Part model, mm, in its own coordinate system. A direction names the side the tool comes from. Round coordinates to 2 decimals unless told otherwise and drop trailing zeros. Loops run counter-clockwise (first coordinate to the right, second up) from the corner with the lowest first, then second, coordinate; pieces in that order, holes last.
1) Drop flat-ended pins along their axis: P1, Ø3, axis at x = 5, z = -2, coming from the -Y side; P2, Ø1, axis at x = 21, z = 2, coming from the +Y side; P3, Ø1.5, axis at x = 39.5, z = 3, coming from the -Y side. Give the stop position or say it passes through.
2) 3-axis set-ups, long thin cutter, end or side, ignore diameter. For faces 1 (the flat face through (-2.19, 0.99, -1.74)), 2 (the flat face through (50, 0, 0)): which of +Z, -Z, +X, -X, +Y, -Y reach the whole face in a straight line?
3) Probe line 1 (Z direction, x = 16.5, y = 0); line 2 (Y direction, x = 7, z = -1.25); line 3 (Y direction, x = 19, z = 2). List the from-to ranges inside material, lowest first.
4) Band-saw the part on A-A, the plane x = 36.5. Write the cut outline in (y, z).
5) Mould opens along Z. For faces 3 (the flat face through (-2, -2, 0)), 4 (the cylindrical face through (24, -3, 0)), 5 (the flat face through (0, -0.1, -3.4)), 6 (the flat face through (-2.186, 1.014, 1.724)) say: +Z half, -Z half, draft (parallel to the pull), parting line (faces both ways), or undercut.
Autodesk Inventor part; units mm, degrees
ref_plane "Work Plane1" through (29, 0, 0) normal (0, -1, 0) x (1, 0, 0)
ref_plane "YZ Plane" through (0, 0, 0) normal (1, 0, 0) x (0, 1, 0)
ref_plane "XZ Plane" through (0, 0, 0) normal (0, 1, 0) x (-1, 0, 0)
sketch "Sketch1" plane through (0, 0, 0) normal (0, 0, 1) x (1, 0, 0)
  line L0 (0.1133, 0) -> (50, 0)
  line L1 (50, 0) -> (50, 3)
  line L2 (50, 3) -> (26, 3)
  line L3 (26, 3) -> (25.3864, 3)
  line L4 (25.3864, 3) -> (0, 3)
  line L5 (0, 3) -> (0, 5.25)
  line L6 (0, 5.25) -> (-3.3, 5.25)
  line L7 (-3.3, 5.25) -> (-3.3, 2.3094)
  line L8 (-3.3, 2.3094) -> (-1.22, 2.3094)
  line L9 (-1.22, 2.3094) -> (0.1133, 0)
  line L10 (-13.96, 0) -> (60.66, 0)
  line L11 (0, -1.05) -> (0, 6.3)
  line L12 (26, 3) -> (0, 3) construction
  dimension "d1" = 24
  dimension "d2" = 0.6136
  dimension "d3" = 3.3
  dimension "d4" = 2.08
  dimension "d5" = 60
  dimension "d6" = 6
  dimension "d7" = 6
  dimension "d8" = 4.6188
  dimension "d9" = 10.5
  dimension "d26" = 50
revolve "Body" add sketch "Sketch1" angle 360 about axis through (0.1133, 0, 0) along (1, 0, 0) contours L9 L11 L4 L3 L2 L1 L0 | L9 L8 L7 L6 L5 L11
sketch "Sketch2" plane through (-3.3, 0, 0) normal (-1, 0, 0) x (0, 0, 1)
  circle A0 centre (0, 0) radius 2.3094
  line L0 (0, -7.35) -> (0, 7.35)
  line L1 (-7.35, 0) -> (7.35, 0)
  line L2 (2.3094, 0) -> (1.1547, -2)
  line L3 (1.1547, -2) -> (-1.1547, -2)
  line L4 (-1.1547, -2) -> (-2.3094, 0)
  line L5 (-2.3094, 0) -> (-1.1547, 2)
  line L6 (-1.1547, 2) -> (1.1547, 2)
  line L7 (1.1547, 2) -> (2.3094, 0)
extrude "Slot" add sketch "Sketch2" against normal up to next contours L7 A0 | A0 L2 | L6 L0 A0 | A0 L0 L3 | L0 L6 A0 | A0 L3 L0 | L4 A0 | A0 L5
fillet "Fillet1" radius 2.56 1 edges at (-3.3, -5.25, 0)
thread "Thread"
chamfer "Chamfer1" distance 0.6135 distance2 0.6135 1 edges at (50, -3, 0) measured on face at (50, -0.7485, -0.2663)
ref_plane "Work Plane1" through (29, 0, 0) normal (0, -1, 0) x (1, 0, 0)
fillet "Fillet2" radius 0.25 1 edges at (0, -3, 0)
equation "\"d1\" = GEL"
equation "\"d3\" = KOH"
equation "\"d4\" = INTI"
equation "\"d6\" = GD"
equation "\"d7\" = BDM"
equation "\"d8\" = 1.1547 * SW"
equation "\"d9\" = KOD"
equation "\"d26\" = NLG"
equation "\"d30\" = R"
equation "\"d17\" = RR"
equation "\"d13\" = GEL"
equation "\"d15\" = -0.5 * SPD + 0.5 * GD"
equation "\"d16\" = GUL"
equation "\"GD\" = NND"
equation "\"NLG\" = 50"
equation "\"GEL\" = 24"
equation "\"KOD\" = 10.5"
equation "\"KOH\" = 3.3"
equation "\"INTI\" = 2.08"
equation "\"GAL\" = 0.61345 * PTC"
equation "\"GUL\" = 0.61345 * PTC"
equation "\"BDM\" = NND"
equation "\"SW\" = 4"
equation "\"RR\" = 2.56"
equation "\"SPD\" = NND - 1.2269 * PTC"
equation "\"R\" = 0.25"
equation "\"TOA\" = 30deg"
equation "\"GD1\" = THREADDIA - 1.2269 * PTC"
equation "\"THREADDIA\" = 6"
equation "\"PTC\" = 1"
equation "\"NND\" = 6"
equation "\"KOH1\" = 0.74"
equation "\"E0\" = 4.583"
properties part number "ISO 7380-1 - M6 x 50" material "Steel"
Reported:
1. P1: stops at y = -2.96
1. P2: stops at y = 2.6
1. P3: stops at y = -1.98
2. face 1: -X
2. face 2: +Z, -Z, +X, +Y, -Y
3. line 1: z = -3 to 3
3. line 2: y = -2.73 to 2.73
3. line 3: y = -2.24 to 2.24
4. outline: circle Ø6 at (0, 0)
5. face 3: undercut
5. face 4: parting line
5. face 5: draft
5. face 6: undercut
